Autodesk Inventor part; units mm, degrees
ref_plane "YZ Plane" through (0, 0, 0) normal (1, 0, 0) x (0, 1, 0)
ref_plane "XZ Plane" through (0, 0, 0) normal (0, 1, 0) x (-1, 0, 0)
ref_plane "XY Plane" through (0, 0, 0) normal (0, 0, 1) x (1, 0, 0)
sketch "Sketch1" plane through (0, 0, 0) normal (1, 0, 0) x (0, 1, 0)
  line L0 (0, 0) -> (-20, 0)
  line L1 (-20, 0) -> (-20, -54.112)
  line L2 (-20, -54.112) -> (0, -54.112)
  line L3 (0, -54.112) -> (0, 0)
  line L4 (-20, 0) -> (-20, -27.056)
  line L5 (-20, -27.056) -> (-20, -34.112)
  line L6 (-20, -34.112) -> (-42, -34.112)
  line L7 (-42, -34.112) -> (-42, -20)
  line L8 (-42, -20) -> (-20, -20)
  line L9 (-20, -20) -> (-20, -34.112)
  line L10 (-20, -20) -> (-18, -20)
  line L11 (-18, -20) -> (-15.5, -20)
  line L12 (-15.5, -20) -> (-15.5, -34.112)
  line L13 (-15.5, -34.112) -> (-18, -34.112)
  line L14 (-18, -34.112) -> (-18, -20)
  line L15 (-20, -20) -> (-20, -15)
  line L16 (-20, -15) -> (-25, -20)
  line L17 (-20, -34.112) -> (-25, -34.112)
  line L18 (-25, -34.112) -> (-20, -39.112)
  line L19 (-20, -34.112) -> (-20, -39.112)
  dimension "d0" = 20
  dimension "d1" = 54.112
  dimension "d2" = 27.056
  dimension "d3" = 7.056
  dimension "d4" = 22
  dimension "d5" = 14.112
  dimension "d6" = 2
  dimension "d7" = 2.5
  dimension "d8" = 5
  dimension "d9" = 45
  dimension "d10" = 5
extrude "Extrusion1" add sketch "Sketch1" along normal blind 2
sketch "Sketch2" plane through (2, 0, 0) normal (1, 0, 0) x (0, 0, -1)
  line L0 (20, -25) -> (20, -42)
  line L1 (34.112, -42) -> (34.112, -25)
  line L2 (20, -25) -> (34.112, -25)
  point P0 (0, 0)
bend part "Bend Part1" radius 3 angle 10 line through (2, -25, -20) along (0, 0, -1) centre toward (-1, 0, 0) moving side (0, -1, 0) both sides no
sketch "Sketch3" plane through (2, 0, 0) normal (1, 0, 0) x (0, 0, -1)
  line L0 (0, 0) -> (0, -20)
  line L1 (0, 0) -> (10, 0)
  line L2 (10, 0) -> (10, -10)
  line L3 (10, -10) -> (0, -10)
  line L4 (0, -10) -> (0, 0)
  line L5 (54.112, 0) -> (0, 0)
  line L6 (54.112, 0) -> (44.112, 0)
  line L7 (44.112, 0) -> (44.112, -10)
  line L8 (44.112, -10) -> (54.112, -10)
  line L9 (54.112, -10) -> (54.112, 0)
  circle A0 centre (10, -10) radius 2.5
  circle A1 centre (44.112, -10) radius 2.5
  dimension "d15" = 10
  dimension "d16" = 10
  dimension "d17" = 10
  dimension "d18" = 10
  dimension "d19" = 5
  dimension "d20" = 5
extrude "Extrusion2" cut sketch "Sketch3" against normal blind 2 contours A0 L2 L3 | L3 L2 A0 | A1 L8 L7 | L7 L8 A1
properties part number "manual_locker_upoper"
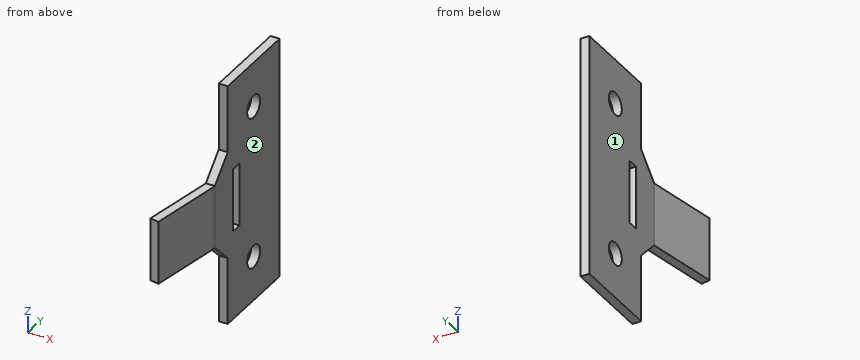
Verification items for the finished model (mm, model axes). Face numbers are marked on the shaded views. A direction names the side the tool comes from. Give positions to 0.01 mm unless a question says otherwise; leave off trailing zeros. Write each loop counter-clockwise with the first axis right and the second up, starting at its lowest first coordinate (ties: lowest second). Pieces come first, ordered by that corner, then holes. Notation, with made-up numbers: M 80.5,60.5 L 130.5,60.5 A23 cw 130.5,93.5 Z; hole C -32.75,5 d7. An arc over 180 degrees is marked long. Write item = value, one per line.
(1) Sectioned sample at B-B (y = -10). Record the cut outline in (x, z), then the cut area to 3 significant figures.
Found:
outline = M 0,-54.11 L 2,-54.11 L 2,-46.61 L 0,-46.61 Z; M 0,-41.61 L 2,-41.61 L 2,-12.5 L 0,-12.5 Z; M 0,-7.5 L 2,-7.5 L 2,0 L 0,0 Z
area = 88.2 mm2
(2) Sectioned sample at D-D (x = 0.75). Record the cut outline in (y, z).
Found:
outline = M -32.35,-34.11 L -25,-34.11 L -20,-39.11 L -20,-54.11 L 0,-54.11 L 0,0 L -20,0 L -20,-15 L -25,-20 L -32.35,-20 Z; hole M -18,-34.11 L -15.5,-34.11 L -15.5,-20 L -18,-20 Z; hole C -10,-44.11 d5; hole C -10,-10 d5
(3) Access from +Z, -Z, +X, -X, +Y, -Y to the whole of each face (thin tool, end or side, straight path). Record for the marked faces 1 and 2.
Found:
face_1 = +Z, -Z, -X, +Y
face_2 = +Z, -Z, +X, +Y, -Y
(4) Material ranges on line 1 (Z direction, x = 0.85, y = -10); line 2 (Y direction, x = 1.5, z = -10); line 3 (Z direction, x = -0.2, y = -36), recorded low to high.
Found:
line_1 = -54.11 to -46.61, -41.61 to -12.5, -7.5 to 0
line_2 = -20 to -12.5, -7.5 to 0
line_3 = -34.11 to -20
(5) Go/stop test with flat-tipped pins: pin 1 Ø12.5 at (y, z) = (-17.5, -23) entering from -X; pin 2 Ø1 at (x, z) = (1.5, -43) entering from -Y; pin 3 Ø2.5 at (x, y) = (0, -35) entering from -Z. Record where each tip stops, or that it passes through.
Found:
pin_1 = 0
pin_2 = -20
pin_3 = -34.11
(6) Sectioned sample at C-C (z = -24). Record the cut outline in (x, y).
Found:
outline = M -2.88,-41.4 L -0.91,-41.75 L 1.95,-25.52 A3 ccw 2,-25 L 2,-18 L 0,-18 L 0,-25 A1 cw -0.02,-25.17 Z; M 0,-15.5 L 2,-15.5 L 2,0 L 0,0 Z
(7) Sectioned sample at A-A (z = -10). Record the cut outline in (x, y), then the cut area to 3 significant figures.
Found:
outline = M 0,-20 L 2,-20 L 2,-12.5 L 0,-12.5 Z; M 0,-7.5 L 2,-7.5 L 2,0 L 0,0 Z
area = 30.0 mm2
